Geometry: final body of the model. Coordinates: model frame, mm. Face numbers are marked on the shaded views. A direction names the side the tool comes from. Round coordinates to 2 decimals unless told otherwise and drop trailing zeros. Loops run counter-clockwise (first coordinate to the right, second up) from the corner with the lowest first, then second, coordinate; pieces in that order, holes last. Notation, with made-up numbers: (44, 53) -> (96, 53) arc R23 cw to (96, 79) -> close; hole circle Ø7 at (-16, 44). An arc over 180 degrees is marked (long way). Answer in a Markdown table with one row per item.
Autodesk Inventor part; units mm, degrees
ref_plane "YZ Plane" through (0, 0, 0) normal (1, 0, 0) x (0, 1, 0)
ref_plane "XZ Plane" through (0, 0, 0) normal (0, 1, 0) x (-1, 0, 0)
ref_plane "XY Plane" through (0, 0, 0) normal (0, 0, 1) x (1, 0, 0)
sketch "Skizze1" plane through (0, 0, 0) normal (1, 0, 0) x (0, 1, 0)
  point P0 (0, 0)
sketch "Skizze2" plane through (0, 0, 0) normal (0, 0, 1) x (1, 0, 0)
  line L0 (0, 0) -> (0, 50)
  ellipse E0 centre (0, 0) end of major axis (0, 50) minor radius 70
  ellipse E1 centre (0, 0) end of major axis (85, 0) minor radius 65
  point P0 (0, 65)
  dimension "d3" = 70
  dimension "d4" = 85
  dimension "d1" = 50
  dimension "d5" = 15
extrude "Extrusion1" add sketch "Skizze2" along normal blind 5
sketch "Skizze4" plane through (0, 0, 5) normal (0, 0, 1) x (1, 0, 0)
  line L0 (-138.5421, 0) -> (141.5539, 0)
  line L1 (141.5539, 0) -> (141.5539, -100.2494)
  line L2 (141.5539, -100.2494) -> (-138.5421, -100.2494)
  line L3 (-138.5421, -100.2494) -> (-138.5421, 0)
extrude "Extrusion3" cut sketch "Skizze4" against normal blind 5
sketch "Skizze5" plane through (0, 0, 5) normal (0, 0, 1) x (1, 0, 0)
  line L0 (-85, 0) -> (-70, 0)
  line L1 (-70, 0) -> (-70, -25)
  line L2 (-70, -25) -> (-85, -25)
  line L3 (-85, -25) -> (-85, 0)
  line L4 (70, 0) -> (85, 0)
  line L5 (85, 0) -> (85, -25)
  line L6 (85, -25) -> (70, -25)
  line L7 (70, -25) -> (70, 0)
  dimension "d13" = 25
  dimension "d14" = 25
extrude "Extrusion4" add sketch "Skizze5" against normal blind 5
sketch "Skizze7" plane through (0, 0, 5) normal (0, 0, 1) x (1, 0, 0)
  line L0 (14.5161, 65.7113) -> (16.129, 65.7113)
  line L1 (16.129, 65.7113) -> (16.129, 66.0339)
  line L2 (16.129, 66.0339) -> (14.5161, 66.0339)
  line L3 (14.5161, 66.0339) -> (14.5161, 65.7113)
  line L4 (-15, 28.2919) -> (15, 28.2919)
  line L5 (15, 28.2919) -> (15, 68.6145)
  line L6 (15, 68.6145) -> (-15, 68.6145)
  line L7 (-15, 68.6145) -> (-15, 28.2919)
  line L8 (-70, -25) -> (-85, -25)
  line L9 (-85, -25) -> (-85, 0)
  ellipse E0 centre (0, 0) end of major axis (-85, 0) minor radius 65 (85, 0) -> (-85, 0) ccw
  line L10 (85, 0) -> (85, -25)
  line L11 (85, -25) -> (70, -25)
  line L12 (70, -25) -> (70, 0)
  ellipse E1 centre (0, 0) end of major axis (-70, 0) minor radius 50 (70, 0) -> (-70, 0) ccw
  line L13 (-70, 0) -> (-70, -25)
  line L14 (0, -43.7229) -> (0, 87.3374)
  dimension "d20" = 30
extrude "Extrusion5" cut sketch "Skizze7" against normal blind 2 contours L3 L2 L5 L0 | L0 L5 E0 L14 L6 L2 L3 | L5 E1 L14 E0 | L5 L4 L14 E1 | L14 E1 L7 E0 | E0 L7 L6 L14 | L14 L4 L7 E1
sketch "Skizze8" plane through (0, 0, 5) normal (0, 0, 1) x (1, 0, 0)
  ellipse E0 centre (0, 0) end of major axis (-85, 0) minor radius 65 (85, 0) -> (15, 63.9799) ccw
  line L0 (0, 0) -> (49.3064, 49.3064) construction
  line L1 (-121.351, 0) -> (133.1061, 0) construction
  line L2 (76.2939, 97.5071) -> (19.9385, 41.1517)
  line L3 (19.9385, 41.1517) -> (41.1517, 19.9385)
  line L4 (41.1517, 19.9385) -> (92.1355, 70.9223)
  line L5 (76.2939, 97.5071) -> (92.1355, 70.9223)
  dimension "d23" = 45
  dimension "d24" = 30
extrude "Extrusion6" cut sketch "Skizze8" against normal blind 2
sketch "Skizze9" plane through (0, 0, 5) normal (0, 0, 1) x (1, 0, 0)
  line L0 (52.5724, 15) -> (140.4, 15)
  line L1 (140.4, 15) -> (140.4, -15)
  line L2 (140.4, -15) -> (52.5724, -15)
  line L3 (52.5724, -15) -> (52.5724, 15)
  line L4 (-125.4, 0) -> (157.4, 0)
  dimension "d27" = 30
extrude "Extrusion7" cut sketch "Skizze9" against normal blind 2
sketch "Skizze10" plane through (0, 0, 5) normal (0, 0, 1) x (1, 0, 0)
  ellipse E0 centre (0, 0) end of major axis (-70, 0) minor radius 50 (-15, 48.8386) -> (-70, 0) ccw
  line L0 (0, 0) -> (-45.6382, 45.6382) construction
  line L1 (-155, 0) -> (125, 0)
  line L2 (-28.1942, 6.981) -> (-6.981, 28.1942)
  line L3 (-6.981, 28.1942) -> (-56.587, 77.8002)
  line L4 (-56.587, 77.8002) -> (-77.8002, 56.587)
  line L5 (-28.1942, 6.981) -> (-77.8002, 56.587)
  dimension "d30" = 45
  dimension "d31" = 30
extrude "Extrusion8" cut sketch "Skizze10" against normal blind 2
sketch "Skizze11" plane through (0, 0, 5) normal (0, 0, 1) x (1, 0, 0)
  ellipse E0 centre (0, 0) end of major axis (-70, 0) minor radius 50 (-53.4768, 32.2636) -> (-70, 0) ccw
  line L0 (-171.6, -15) -> (-171.6, 15)
  line L1 (-171.6, 15) -> (-38.4, 15)
  line L2 (-38.4, 15) -> (-38.4, -15)
  line L3 (-38.4, -15) -> (-171.6, -15)
  line L4 (-188.6, 0) -> (130.6, 0)
  dimension "d34" = 30
extrude "Extrusion9" cut sketch "Skizze11" against normal blind 2
sketch "Skizze12" plane through (0, 0, 3) normal (0, 0, 1) x (1, 0, 0)
  ellipse E0 centre (0, 0) end of major axis (-70, 0) minor radius 50 (15, 48.8386) -> (-15, 48.8386) ccw
  line L0 (-15, 48.8386) -> (-15, 63.9799)
  line L1 (-7.5, 49.7122) -> (-7.5, 23.0205)
  line L2 (0, -43) -> (0, 83) construction
  line L3 (7.5, 49.7122) -> (7.5, 23.0205)
  line L4 (-7.5, 23.0205) -> (-70, -8.2295)
  line L5 (-70, 0) -> (-70, -15) construction
  line L6 (7.5, 23.0205) -> (70, -8.2295)
  line L7 (70, -15) -> (70, 0) construction
  line L8 (-70, -8.2295) -> (-70, -25)
  line L9 (70, -25) -> (70, -8.2295)
  line L10 (-7.5, 49.7122) -> (0, 53)
  line L11 (0, 53) -> (7.5, 49.7122)
  line L12 (0, 10) -> (-70, -25)
  line L13 (0, 10) -> (70, -25)
  dimension "d37" = 15
  dimension "d41" = 53
  dimension "d43" = 15
  dimension "d44" = 15
  dimension "d45" = 10
extrude "Extrusion10" add sketch "Skizze12" against normal blind 3
properties part number "Laseraufbau"
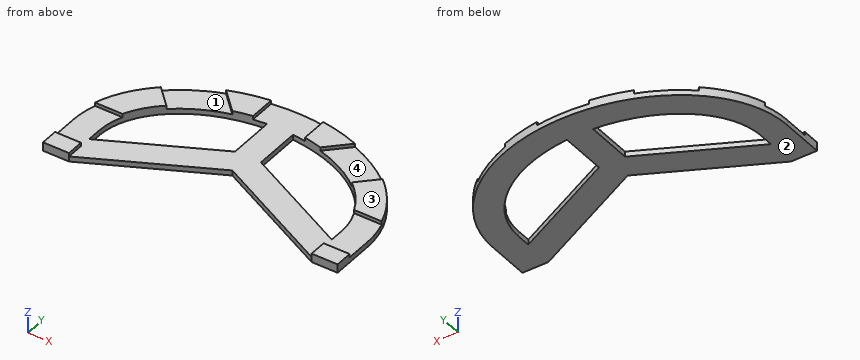
Item 1: Reachability of the marked faces 1 and 2 from +Z, -Z, +X, -X, +Y, -Y: full face, straight path, thin tool, end or side. Return the list, or none.
Answer:
| item | result |
|---|---|
| face 1 | +Z |
| face 2 | -Z, +X, -X, +Y, -Y |
Item 2: Line query: probe 1 along X at (y, z) = (1.5, 0.7); probe 2 along X at (y, z) = (29, 2.75); probe 3 along X at (y, z) = (0.5, 2). Output: solid intervals per line, ascending. Write a range as [from, to].
Answer:
| item | result |
|---|---|
| probe 1 | x = [-84.98, -69.97], [-50.54, -17], [17, 50.54], [69.97, 84.98] |
| probe 2 | x = [-76.07, -57.02], [-7.5, 7.5], [57.02, 76.07] |
| probe 3 | x = [-85, -70], [-52.54, -19], [19, 52.54], [70, 85] |
Item 3: Pin query (flat end, axial travel): pin 1 Ø2 at (y, z) = (56.5, 3.5) entering from +X; pin 2 Ø8 at (x, y) = (-33, 47.5) entering from +Z; pin 3 Ø1 at (x, z) = (-74, 4) entering from +Y. Return the tip coordinate at first contact, or that it passes through.
Answer:
| item | result |
|---|---|
| pin 1 | stops at x = 43.96 |
| pin 2 | stops at z = 3 |
| pin 3 | stops at y = 32.65 |
Item 4: Cut plane A-A (y = -19). Output: boundary loops of the cut face in (x, z), then the cut area to 3 significant figures.
Answer:
| item | result |
|---|---|
| outline | (-85, 0) -> (-58, 0) -> (-58, 3) -> (-70, 3) -> (-70, 5) -> (-85, 5) -> close; (58, 0) -> (85, 0) -> (85, 5) -> (70, 5) -> (70, 3) -> (58, 3) -> close |
| area | 222 mm² |
Item 5: Draft query along X for the marked faces 3 and 4. Return one class per face: pulls with the +X half, pulls with the -X half, needs draft (parallel to the pull), parting line crosses it, or undercut.
Answer:
| item | result |
|---|---|
| face 3 | needs draft |
| face 4 | undercut |
Item 6: Cut plane B-B (z = 4.15). Count the separate pieces of the cut face and the enclosed holes in it, then the cut area to 3 significant figures.
Answer:
| item | result |
|---|---|
| separate pieces | 6 |
| enclosed holes | 0 |
| area | 1,640 mm² |
